Could you check a few things on this drawing? It's one solid part, dimensions in mm from its lowest x, y, z. Round coordinates to 2 decimals unless told otherwise and drop trailing zeros. Loops run counter-clockwise (first coordinate to the right, second up) from the corner with the lowest first, then second, coordinate; pieces in that order, holes last. Notation, with made-up numbers: (59, -28.5) -> (70, -28.5) arc R18 cw to (70, -11.5) -> close; hole circle Ø2 at (-5.75, 23.25). An arc over 180 degrees is marked (long way). Use one line per item in the form item = value. Start each with the question number.
Item 1: Thinking about a two-plate mould opening in Y: for the marked faces 1, 2 and 3, which applies, released by +Y, released by -Y, zero draft, split by the parting line, or undercut?
Item 2: If we section it at D-D (z = 5.75): Write out the boundary of the cut face in (x, y), then the cut area to 3 significant figures.
Item 3: If we section it at A-A (x = 20.25): Write out the boundary of the cut face in (y, z), then the cut area to 4 significant figures.
Item 4: If I drill on L1, parallel to Y at x = 20.25, z = 4.5; L2, parallel to X at y = 4.1, z = 4.75; L3, parallel to X at y = 1.9, z = 2.75, over which ranges is the centre line in solid material (lowest first)? Write a range as [from, to].
Item 5: If we section it at B-B (z = 1): Write out the boundary of the cut face in (x, y), then the cut area to 3 significant figures.
Item 6: I'm going to push a flat-ended pin straight in: pin 1 Ø1.8 at (x, y) = (2.75, 2.75) entering from +Z. Where does the tip first touch, or does it pass through?
Item 7: If we section it at C-C (y = 2.75): Write out the boundary of the cut face in (x, z), then the cut area to 3 significant figures.
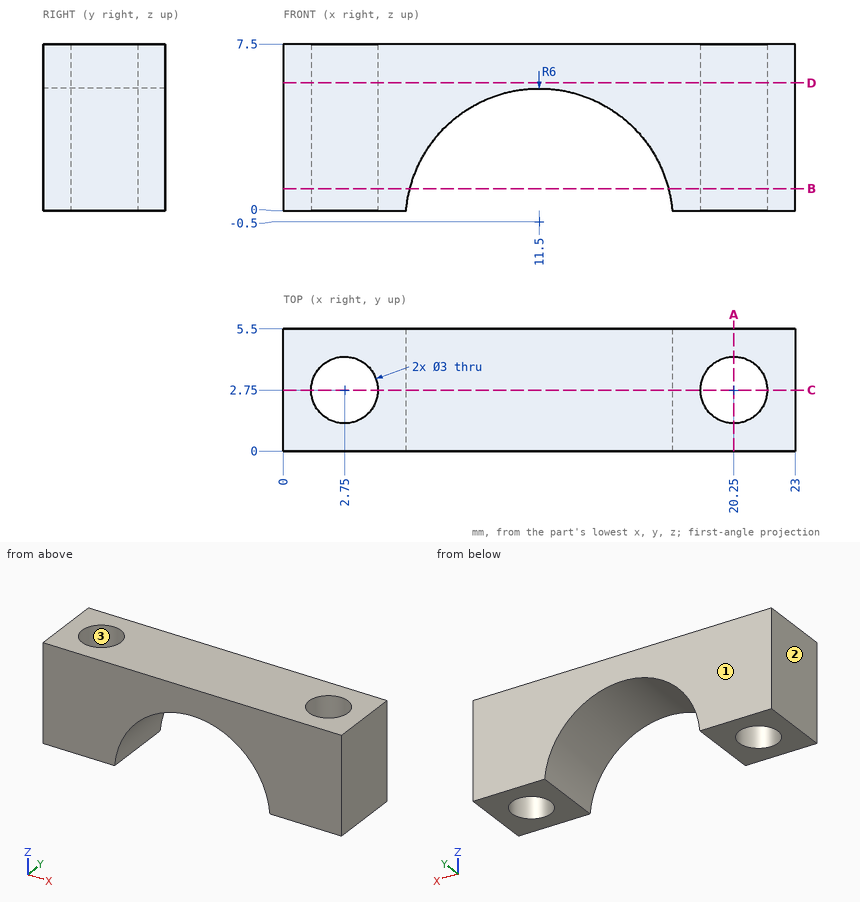
Values found:
q1.face_1 = released by +Y
q1.face_2 = zero draft
q1.face_3 = undercut
q2.outline = (0, 0) -> (23, 0) -> (23, 5.5) -> (0, 5.5) -> close; hole circle Ø3 at (2.75, 2.75); hole circle Ø3 at (20.25, 2.75)
q2.area = 112 mm2
q3.outline = (0, 0) -> (1.25, 0) -> (1.25, 7.5) -> (0, 7.5) -> close; (4.25, 0) -> (5.5, 0) -> (5.5, 7.5) -> (4.25, 7.5) -> close
q3.area = 18.75 mm2
q4.L1 = [0, 1.25], [4.25, 5.5]
q4.L2 = [0, 2.1], [3.4, 8.6], [14.4, 19.6], [20.9, 23]
q4.L3 = [0, 1.51], [3.99, 6.46], [16.54, 19.01], [21.49, 23]
q5.outline = (0, 0) -> (5.69, 0) -> (5.69, 5.5) -> (0, 5.5) -> close; (17.31, 0) -> (23, 0) -> (23, 5.5) -> (17.31, 5.5) -> close; hole circle Ø3 at (2.75, 2.75); hole circle Ø3 at (20.25, 2.75)
q5.area = 48.5 mm2
q6.pin_1 = through
q7.outline = (0, 0) -> (1.25, 0) -> (1.25, 7.5) -> (0, 7.5) -> close; (4.25, 0) -> (5.52, 0) arc R6 cw to (17.48, 0) -> (18.75, 0) -> (18.75, 7.5) -> (4.25, 7.5) -> close; (21.75, 0) -> (23, 0) -> (23, 7.5) -> (21.75, 7.5) -> close
q7.area = 76.9 mm2
